Autodesk Inventor part; units mm, degrees
ref_plane "YZ Plane" through (0, 0, 0) normal (1, 0, 0) x (0, 1, 0)
ref_plane "XZ Plane" through (0, 0, 0) normal (0, 1, 0) x (-1, 0, 0)
ref_plane "XY Plane" through (0, 0, 0) normal (0, 0, 1) x (1, 0, 0)
sketch "Sketch1" plane through (0, 0, 0) normal (0, 1, 0) x (-1, 0, 0)
  line L0 (0, 0) -> (-15, 0)
  line L1 (-15, 0) -> (-15, -68)
  line L2 (-15, -68) -> (0, -68)
  line L3 (0, -68) -> (0, 0)
  dimension "d0" = 15
  dimension "d1" = 68
extrude "Extrusion1" add sketch "Sketch1" along normal blind 16
sketch "Sketch2" plane through (15, 0, 0) normal (1, 0, 0) x (0, 0, -1)
  line L0 (34.4, 3.375) -> (29.4, 3.375)
  line L1 (34.4, 13.119) -> (29.4, 13.119)
  line L2 (0, 0) -> (0, 16)
  line L3 (29.4, 13.119) -> (0, 13.119)
  line L4 (0, 13.119) -> (0, 3.375)
  line L5 (0, 3.375) -> (29.4, 3.375)
  line L6 (29.4, 3.375) -> (29.4, 13.119)
extrude "Extrusion2" add sketch "Sketch2" along normal up to surface (5.25 mm away)
properties part number "smolLipo"
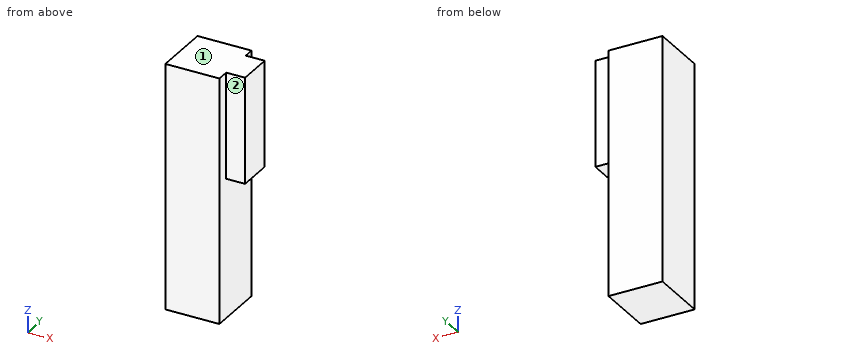
Design review of the part built by this model. Coordinates are the model's own, in mm. Face numbers are marked on the shaded views. A direction names the side the tool comes from. Coordinates: 2 decimals unless noted, no trailing zeros. Write each loop counter-clockwise with the first axis right and the second up, starting at its lowest first coordinate (ties: lowest second). Pieces come first, ordered by that corner, then holes. Notation, with made-up numbers: (36.5, 78.25) -> (68.5, 78.25) arc R32 cw to (68.5, 113.25) -> close; hole circle Ø1 at (43.25, -28.5). An arc over 180 degrees is marked (long way). Write each question's results on one line, items separated by ' | '. Start each with the question number.
(1) Tool access review of the marked faces 1 and 2: name each direction out of +Z, -Z, +X, -X, +Y, -Y from which nothing blocks a thin tool from reaching the whole face with its end or side.
(2) For line 1 along Y through (x, z) = (19, -27) (3 decimals); line 2 along Z through (x, y) = (17.75, 6.75); line 3 along X through (y, z) = (12.5, -31.5), list the stretches that pass through material, from the lowest coordinate up. Write a range as from..to.
(3) Take a section at A-A on z = -11.5. Write out the cut boundary in (x, y) (3 decimals).
(4) Clearance check with flat-ended pins moving along their axes: P1, Ø2, axis at x = 18, z = -26, coming from the +Y side; P2, Ø2.5, axis at x = 16.5, z = -16.5, coming from the -Y side (3 decimals). State where each tip first meets the part, or that it passes through.
(5) Take a section at C-C on x = 16.5. Write out the cut boundary in (y, z) (3 decimals), and give its area (3 significant figures).
(6) Take a section at B-B on y = 7. Write out the cut boundary in (x, z).
(7) Take a section at D-D on y = 14.75. Write out the cut boundary in (x, z), and give its area (3 significant figures).
Results found:
1) face 1: +Z, +X, -X, +Y, -Y | face 2: +Z, -Z, +X, -Y
2) line 1: y = 3.375..13.119 | line 2: z = -29.4..0 | line 3: x = 0..15
3) outline: (0, 0) -> (15, 0) -> (15, 3.375) -> (20.25, 3.375) -> (20.25, 13.119) -> (15, 13.119) -> (15, 16) -> (0, 16) -> close
4) P1: stops at y = 13.12 | P2: stops at y = 3.375
5) outline: (3.375, -29.4) -> (13.119, -29.4) -> (13.119, 0) -> (3.375, 0) -> close | area: 286 mm2
6) outline: (0, -68) -> (15, -68) -> (15, -29.4) -> (20.25, -29.4) -> (20.25, 0) -> (0, 0) -> close
7) outline: (0, -68) -> (15, -68) -> (15, 0) -> (0, 0) -> close | area: 1,020 mm2
